Part model, mm, in its own coordinate system. A direction names the side the tool comes from. Coordinates: 2 decimals unless noted, no trailing zeros. Write each loop counter-clockwise with the first axis right and the second up, starting at its lowest first coordinate (ties: lowest second). Pieces come first, ordered by that corner, then holes. Notation, with made-up numbers: (-38, 52.25) - (-27, 52.25) arc R4 cw to (-27, 58.25) - close; hole circle Ø2 at (25, 53). An arc over 180 degrees is marked (long way). Use a Markdown table: item, result.
```python
from build123d import *

# Parameters (mm, degrees)
SKETCH_1_R             = 13
SKETCH_1_R_2           = 2.6
SM_BASE_FLANGE_1_DEPTH = 2


# Sheet-metal steps are written as plain solids
with BuildPart() as part:
    # Sketch 1 → 基体-法兰1 (new body)
    with BuildSketch(Plane.XY):
        with BuildLine():
            Line((42, 18), (42, -18))
            ThreePointArc((42, -18), (41.121320344, -20.121320344), (39, -21))
            Line((39, -21), (-18, -21))
            ThreePointArc((-18, -21), (-20.121320344, -20.121320344), (-21, -18))
            Line((-21, -18), (-21, 18))
            ThreePointArc((-21, 18), (-20.121320344, 20.121320344), (-18, 21))
            Line((-18, 21), (39, 21))
            ThreePointArc((39, 21), (41.121320344, 20.121320344), (42, 18))
        make_face()
        Circle(SKETCH_1_R, mode=Mode.SUBTRACT)
        with Locations((32, 15)):
            Circle(SKETCH_1_R_2, mode=Mode.SUBTRACT)
        with Locations((32, -15)):
            Circle(SKETCH_1_R_2, mode=Mode.SUBTRACT)
        with BuildLine():
            Line((-14, 13.9), (-17, 13.9))
            ThreePointArc((-17, 13.9), (-18.6, 15.5), (-17, 17.1))
            Line((-17, 17.1), (-14, 17.1))
            ThreePointArc((-14, 17.1), (-12.4, 15.5), (-14, 13.9))
        make_face(mode=Mode.SUBTRACT)
        with BuildLine():
            Line((-14, -17.1), (-17, -17.1))
            ThreePointArc((-17, -17.1), (-18.6, -15.5), (-17, -13.9))
            Line((-17, -13.9), (-14, -13.9))
            ThreePointArc((-14, -13.9), (-12.4, -15.5), (-14, -17.1))
        make_face(mode=Mode.SUBTRACT)
        with BuildLine():
            Line((17, 13.9), (14, 13.9))
            ThreePointArc((14, 13.9), (12.4, 15.5), (14, 17.1))
            Line((14, 17.1), (17, 17.1))
            ThreePointArc((17, 17.1), (18.6, 15.5), (17, 13.9))
        make_face(mode=Mode.SUBTRACT)
        with BuildLine():
            Line((17, -17.1), (14, -17.1))
            ThreePointArc((14, -17.1), (12.4, -15.5), (14, -13.9))
            Line((14, -13.9), (17, -13.9))
            ThreePointArc((17, -13.9), (18.6, -15.5), (17, -17.1))
        make_face(mode=Mode.SUBTRACT)
    extrude(amount=-SM_BASE_FLANGE_1_DEPTH)


solid = part.part
```
Item 1: Band-saw the part on C-C, the plane y = 15. Give the cut face in (x, z).
From the geometry:
| item | result |
|---|---|
| outline | (-21, -2) - (-18.52, -2) - (-18.52, 0) - (-21, 0) - close; (-12.48, -2) - (12.48, -2) - (12.48, 0) - (-12.48, 0) - close; (18.52, -2) - (29.4, -2) - (29.4, 0) - (18.52, 0) - close; (34.6, -2) - (42, -2) - (42, 0) - (34.6, 0) - close |
Item 2: Drill centre lines: probe 1 along Y at (x, z) = (32, -0.45); probe 2 along Y at (x, z) = (0, -0.5); probe 3 along Y at (x, z) = (33.5, -0.8). Where is each one in solid material? Low to high.
From the geometry:
| item | result |
|---|---|
| probe 1 | -21 to -17.6, -12.4 to 12.4, 17.6 to 21 |
| probe 2 | -21 to -13, 13 to 21 |
| probe 3 | -21 to -17.12, -12.88 to 12.88, 17.12 to 21 |
Item 3: Band-saw the part on D-D, the plane y = 7.5. Give the cut face in (x, z).
From the geometry:
| item | result |
|---|---|
| outline | (-21, -2) - (-10.62, -2) - (-10.62, 0) - (-21, 0) - close; (10.62, -2) - (42, -2) - (42, 0) - (10.62, 0) - close |
Item 4: Two-plate mould, pull along Y, no slides. Class faces 3 (the face through (-18.6, 15.5, -1)), 4 (the face through (41.14, -20.1, -0.99)), 5 (the face through (-20.14, 20.1, -0.99)): pulls with the +Y half, pulls with the -Y half, needs draft (parallel to the pull), parting line crosses it, or undercut.
From the geometry:
| item | result |
|---|---|
| face 3 | undercut |
| face 4 | pulls with the -Y half |
| face 5 | pulls with the +Y half |
Item 5: Band-saw the part on B-B, the plane y = 0. Give the cut face in (x, z).
From the geometry:
| item | result |
|---|---|
| outline | (-21, -2) - (-13, -2) - (-13, 0) - (-21, 0) - close; (13, -2) - (42, -2) - (42, 0) - (13, 0) - close |
Item 6: Band-saw the part on A-A, the plane z = -0.55. Give the cut face in (x, y), then the cut area to 3 significant figures.
From the geometry:
| item | result |
|---|---|
| outline | (-21, -18) arc R3 ccw to (-18, -21) - (39, -21) arc R3 ccw to (42, -18) - (42, 18) arc R3 ccw to (39, 21) - (-18, 21) arc R3 ccw to (-21, 18) - close; hole (-17, -17.1) - (-14, -17.1) arc R1.6 ccw to (-14, -13.9) - (-17, -13.9) arc R1.6 ccw to start; hole (-17, 13.9) - (-14, 13.9) arc R1.6 ccw to (-14, 17.1) - (-17, 17.1) arc R1.6 ccw to start; hole circle Ø26 at (0, 0); hole (14, -17.1) - (17, -17.1) arc R1.6 ccw to (17, -13.9) - (14, -13.9) arc R1.6 ccw to start; hole (14, 13.9) - (17, 13.9) arc R1.6 ccw to (17, 17.1) - (14, 17.1) arc R1.6 ccw to start; hole circle Ø5.2 at (32, -15); hole circle Ø5.2 at (32, 15) |
| area | 1,990 mm^2 |
Item 7: Which spindle directions (+Z, -Z, +X, -X, +Y, -Y) get a long thin tool onto all of the face, cutting with end or side? Do faces 1 (the face through (16, -17.1, -1)), 2 (the face through (-20.1, -20.14, -0.99)). Say none if no direction does.
From the geometry:
| item | result |
|---|---|
| face 1 | +Z, -Z |
| face 2 | +Z, -Z, -X, -Y |
